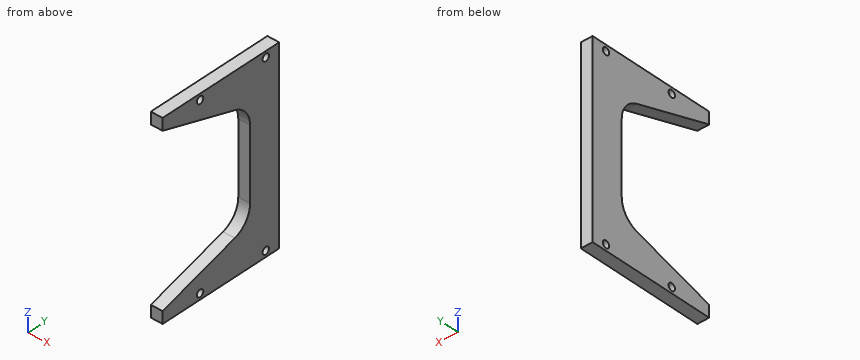
```python
from build123d import *

# Parameters (mm, degrees)
BOSS_EXTRUDE1_DEPTH       = 6.35
F_6_CLEARANCE_HOLE1_D     = 3.7973
F_6_CLEARANCE_HOLE1_DEPTH = 9.398
F_6_CLEARANCE_HOLE1_TIP   = 1.140824014


with BuildPart() as part:
    # Sketch1 → Boss-Extrude1 (new body)
    with BuildSketch(Plane.ZY.offset(60.933137827)):
        Polygon((-95.039403682, -15.875), (-95.039403682, 46.928467802), (-6.35, 46.928467802), (-6.35, -15.875), (0, -15.875), (0, 53.278467802), (-101.389403682, 53.278467802), (-101.389403682, -15.875), align=None)
        with BuildLine():
            Line((-6.35, 46.928467802), (-95.039403682, 46.928467802))
            Line((-95.039403682, 46.928467802), (-95.039403682, -15.875))
            Line((-95.039403682, -15.875), (-82.154349913, 26.960143079))
            ThreePointArc((-82.154349913, 26.960143079), (-77.569908616, 33.493757292), (-69.992656184, 36.001836689))
            Line((-69.992656184, 36.001836689), (-31.396747499, 36.001836689))
            ThreePointArc((-31.396747499, 36.001836689), (-23.819495066, 33.493757292), (-19.23505377, 26.960143079))
            Line((-19.23505377, 26.960143079), (-6.35, -15.875))
            Line((-6.35, -15.875), (-6.35, 46.928467802))
        make_face()
    extrude(amount=BOSS_EXTRUDE1_DEPTH)

    # #6 Clearance Hole1
    with Locations(Plane.ZY.offset(67.283137827)):
        with Locations((-3.175, 45.340967802), (-3.175, 6.35), (-98.214403682, 6.35), (-98.214403682, 45.340967802)):
            Hole(F_6_CLEARANCE_HOLE1_D / 2, depth=F_6_CLEARANCE_HOLE1_DEPTH)
            with Locations((0, 0, -(F_6_CLEARANCE_HOLE1_DEPTH + F_6_CLEARANCE_HOLE1_TIP / 2))):  # 118° drill point
                Cone(0, F_6_CLEARANCE_HOLE1_D / 2, F_6_CLEARANCE_HOLE1_TIP, mode=Mode.SUBTRACT)


solid = part.part
```
Work out the finished part from the listing and answer in its coordinate system (mm). Give positions to 0.01 mm unless a question says otherwise; leave off trailing zeros. Write each loop counter-clockwise with the first axis right and the second up, starting at its lowest first coordinate (ties: lowest second). Pieces come first, ordered by that corner, then holes. Notation, with made-up numbers: (46, 83.25) -> (72, 83.25) arc R24 cw to (72, 117.25) -> close; hole circle Ø4 at (61.25, 80.5). An arc over 180 degrees is marked (long way). Write each question's results on one line, items separated by ' | '.
1. Straight lines are drawn through the part: L1, parallel to Z at x = -62.75, y = 27; L2, parallel to Y at x = -61.5, z = -42; L3, parallel to Z at x = -62, y = -2. For each, find the intervals that lie inside material, in ascending order.
Data:
L1: -101.39 to -82.14, -19.25 to 0 | L2: 36 to 53.28 | L3: -101.39 to -90.87, -10.52 to 0
2. Each of these flat-tipped pins is pushed along its axis until it touches: pin 1 Ø5 at (y, z) = (6.35, -3.175) entering from -X; pin 2 Ø1.5 at (x, z) = (-65.5, -45) entering from -Y. Where does it stop, or does it pass through?
Data:
pin 1: x = -67.28 | pin 2: y = 36
3. Find section C-C on z = -48. Determine the outline of the cut face in (x, y).
Data:
outline: (-67.28, 36) -> (-60.93, 36) -> (-60.93, 53.28) -> (-67.28, 53.28) -> close
4. Find section D-D on x = -65. Determine the outline of the cut face in (y, z) (3 decimals), and give its area (3 significant figures).
Data:
outline: (-15.875, -101.389) -> (53.278, -101.389) -> (53.278, 0) -> (-15.875, 0) -> (-15.875, -6.35) -> (26.96, -19.235) arc R12.7 cw to (36.002, -31.397) -> (36.002, -69.993) arc R12.7 cw to (26.96, -82.154) -> (-15.875, -95.039) -> close; hole circle Ø3.797 at (6.35, -98.214); hole circle Ø3.797 at (6.35, -3.175); hole circle Ø3.797 at (45.341, -98.214); hole circle Ø3.797 at (45.341, -3.175) | area: 3,210 mm^2
5. Find section B-B on y = 6.35. Determine the outline of the cut face in (x, z), and give its area (3 significant figures).
Data:
outline: (-67.28, -101.39) -> (-60.93, -101.39) -> (-60.93, -100.11) -> (-67.28, -100.11) -> close; (-67.28, -96.32) -> (-60.93, -96.32) -> (-60.93, -88.35) -> (-67.28, -88.35) -> close; (-67.28, -13.04) -> (-60.93, -13.04) -> (-60.93, -5.07) -> (-67.28, -5.07) -> close; (-67.28, -1.28) -> (-60.93, -1.28) -> (-60.93, 0) -> (-67.28, 0) -> close | area: 117 mm^2
6. Find section A-A on y = 34. Determine the outline of the cut face in (x, z), and give its area (3 significant figures).
Data:
outline: (-67.28, -101.39) -> (-60.93, -101.39) -> (-60.93, -76.84) -> (-67.28, -76.84) -> close; (-67.28, -24.55) -> (-60.93, -24.55) -> (-60.93, 0) -> (-67.28, 0) -> close | area: 312 mm^2
